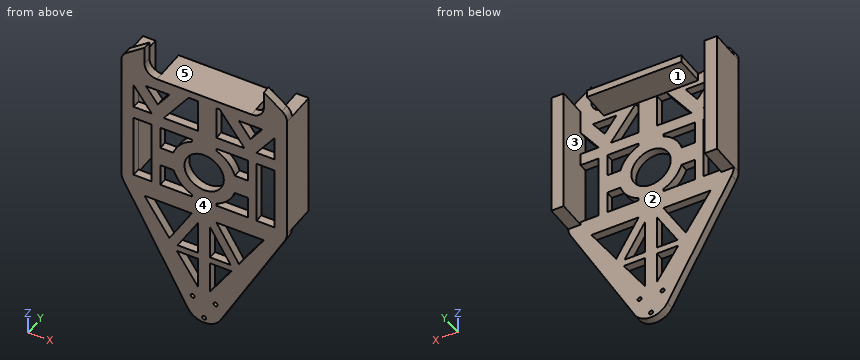
```python
from build123d import *

# Parameters (mm, degrees)
SKETCH1_R            = 47.5
BOSS_EXTRUDE6_DEPTH  = 20
FILLET2_R            = 30
SKETCH3_W            = 227.888974491
SKETCH3_H            = 17.82820952
SKETCH3_W_2          = 30.029703607
SKETCH3_H_2          = 306.819916415
SKETCH3_W_3          = 30
BOSS_EXTRUDE12_DEPTH = 70
FILLET3_R            = 45
FILLET4_R            = 45
SKETCH4_R            = 4.852465173
CUT_EXTRUDE2_DEPTH   = 21


with BuildPart() as part:
    # Sketch1 → Boss-Extrude6 (new body)
    with BuildSketch(Plane(origin=(0, 0, 0), x_dir=(1, 0, 0), z_dir=(0, 1, 0))):
        Polygon((-324.500042801, -72.630227613), (-324.500042801, 0), (-36.61106831, 0), (-36.61106831, -72.630227613), (19.444444444, -30.98937664), (19.444444444, 0), (19.444444444, 300), (-180.555555556, 662.976241067), (-380.555555556, 300), (-380.555555556, 0), (-380.555555556, -30.98937664), align=None)
        Polygon((-264.055692307, 30), (-320.898350202, 30), (-292.477021255, 68.259836918), align=None, mode=Mode.SUBTRACT)
        Polygon((-350.555555556, 40.384990781), (-350.555555556, 98.955926659), (-307.046121917, 98.955926659), align=None, mode=Mode.SUBTRACT)
        Polygon((-194.895952536, 18.381237109), (-218.052993309, 18.381237109), (-277.907920592, 98.955926659), (-194.895952536, 98.955926659), align=None, mode=Mode.SUBTRACT)
        Polygon((-307.046121917, 128.955926659), (-350.555555556, 128.955926659), (-350.555555556, 178.791030317), (-350.555555556, 221.457829656), (-350.555555556, 283.955926659), (-307.046121917, 283.955926659), (-307.046121917, 221.457829656), (-307.046121917, 178.791030317), align=None, mode=Mode.SUBTRACT)
        with BuildLine():
            Line((-210.32776095, 128.955926659), (-286.18247229, 128.955926659))
            Line((-286.18247229, 128.955926659), (-286.18247229, 183.722078004))
            Line((-286.18247229, 183.722078004), (-254.646190087, 183.722078004))
            ThreePointArc((-254.646190087, 183.722078004), (-237.937656941, 154.364234033), (-210.32776095, 134.902689235))
            Line((-210.32776095, 134.902689235), (-210.32776095, 128.955926659))
        make_face(mode=Mode.SUBTRACT)
        with BuildLine():
            Line((-286.18247229, 230.610640855), (-286.18247229, 283.955926659))
            Line((-286.18247229, 283.955926659), (-210.32776095, 283.955926659))
            Line((-210.32776095, 283.955926659), (-210.32776095, 278.009164084))
            ThreePointArc((-210.32776095, 278.009164084), (-237.43400989, 259.09708387), (-254.195217302, 230.610640855))
            Line((-254.195217302, 230.610640855), (-286.18247229, 230.610640855))
        make_face(mode=Mode.SUBTRACT)
        with Locations((-180.555555556, 206.455926659)):
            Circle(SKETCH1_R, mode=Mode.SUBTRACT)
        Polygon((-143.058117802, 18.381237109), (-150.783350161, 18.381237109), (-150.783350161, 98.955926659), (-83.203190519, 98.955926659), align=None, mode=Mode.SUBTRACT)
        Polygon((-68.634089856, 68.259836918), (-40.212760909, 30), (-97.055418804, 30), align=None, mode=Mode.SUBTRACT)
        Polygon((-10.555555556, 98.955926659), (-10.555555556, 40.384990781), (-54.064989194, 98.955926659), align=None, mode=Mode.SUBTRACT)
        with BuildLine():
            Line((-150.783350161, 128.955926659), (-150.783350161, 134.902689235))
            ThreePointArc((-150.783350161, 134.902689235), (-123.17345417, 154.364234033), (-106.464921024, 183.722078004))
            Line((-106.464921024, 183.722078004), (-74.928638821, 183.722078004))
            Line((-74.928638821, 183.722078004), (-74.928638821, 128.955926659))
            Line((-74.928638821, 128.955926659), (-150.783350161, 128.955926659))
        make_face(mode=Mode.SUBTRACT)
        with BuildLine():
            ThreePointArc((-106.915893809, 230.610640855), (-123.677101221, 259.09708387), (-150.783350161, 278.009164084))
            Line((-150.783350161, 278.009164084), (-150.783350161, 283.955926659))
            Line((-150.783350161, 283.955926659), (-74.928638821, 283.955926659))
            Line((-74.928638821, 283.955926659), (-74.928638821, 230.610640855))
            Line((-74.928638821, 230.610640855), (-106.915893809, 230.610640855))
        make_face(mode=Mode.SUBTRACT)
        Polygon((-10.555555556, 178.791030317), (-10.555555556, 128.955926659), (-54.064989194, 128.955926659), (-54.064989194, 178.791030317), (-54.064989194, 221.457829656), (-54.064989194, 283.955926659), (-10.555555556, 283.955926659), (-10.555555556, 221.457829656), align=None, mode=Mode.SUBTRACT)
        Polygon((-210.32776095, 330), (-324.500042801, 330), (-264.477795432, 420.033371054), align=None, mode=Mode.SUBTRACT)
        Polygon((-194.895952536, 348.542048906), (-244.539447118, 431.082553467), (-194.895952536, 431.082553467), align=None, mode=Mode.SUBTRACT)
        Polygon((-246.308768225, 447.286911864), (-194.895952536, 524.406135398), (-194.895952536, 447.286911864), align=None, mode=Mode.SUBTRACT)
        Polygon((-96.633315679, 420.033371054), (-36.61106831, 330), (-150.783350161, 330), align=None, mode=Mode.SUBTRACT)
        Polygon((-166.215158575, 431.082553467), (-116.571663993, 431.082553467), (-166.215158575, 348.542048906), align=None, mode=Mode.SUBTRACT)
        Polygon((-166.215158575, 524.406135398), (-114.802342886, 447.286911864), (-166.215158575, 447.286911864), align=None, mode=Mode.SUBTRACT)
    extrude(amount=BOSS_EXTRUDE6_DEPTH)

    # Fillet2
    fillet2_edges = [part.edges().sort_by_distance(p)[0] for p in [
        (19.444444444, 10, 30.98937664),
        (-36.61106831, 10, 0),
        (-324.500042801, 10, 0),
        (-380.555555556, 10, 30.98937664),
    ]]
    fillet(fillet2_edges, radius=FILLET2_R)

    # Sketch3 → Boss-Extrude12 (add)
    with BuildSketch(Plane(origin=(0, 20, 0), x_dir=(1, 0, 0), z_dir=(0, 1, 0))):
        with Locations((-180.555555556, 8.91410476)):
            Rectangle(SKETCH3_W, SKETCH3_H)
        with Locations((-365.540703753, 137.50677266)):
            Rectangle(SKETCH3_W_2, SKETCH3_H_2)
        with Locations((4.444444444, 137.50677266)):
            Rectangle(SKETCH3_W_3, SKETCH3_H_2)
    extrude(amount=BOSS_EXTRUDE12_DEPTH)

    # Fillet3
    fillet3_edges = [part.edges().sort_by_distance(p)[0] for p in [
        (-180.555555556, 10, -662.976241067),
    ]]
    fillet(fillet3_edges, radius=FILLET3_R)

    # Fillet4
    fillet4_edges = [part.edges().sort_by_distance(p)[0] for p in [
        (-380.555555556, 10, -300),
        (19.444444444, 10, -300),
    ]]
    fillet(fillet4_edges, radius=FILLET4_R)

    # Sketch4 → Cut-Extrude2 (cut, through all)
    with BuildSketch(Plane(origin=(0, 20, 0), x_dir=(1, 0, 0), z_dir=(0, 1, 0))):
        with Locations((-180.555555556, 601.729619553)):
            Circle(SKETCH4_R)
        with Locations((-208.268368477, 553.729619553)):
            Circle(SKETCH4_R)
        with Locations((-152.842742634, 553.729619553)):
            Circle(SKETCH4_R)
    extrude(amount=-CUT_EXTRUDE2_DEPTH, mode=Mode.SUBTRACT)


solid = part.part
```
The listing builds one solid part. Answer for the finished solid, in the listing's coordinates (mm). Face numbers are marked on the shaded views. A direction names the side the tool comes from. Give positions to 0.01 mm unless a question says otherwise; leave off trailing zeros. Order: outer loops, then holes, each group sorted by start corner. A loop starts at its lowest first (then second) coordinate and runs counter-clockwise, first axis right, second up. Notation, with made-up numbers: (-1, 31.25) - (39, 31.25) arc R28 ccw to (39, 52.25) - close; hole circle Ø1 at (52.5, 25.5). An arc over 180 degrees is marked (long way). Answer in a Markdown table with one row per item. Add a question column.
Q1. Which of the six approach directions +Z, -Z, +X, -X, +Y, -Y give full straight-line access (tool end or side, diameter ignored) to the marked faces 4 and 5?
Q2. The part is cut by section B-B (z = -486.5). Determine the outline of the cut face in (x, y).
Q3. For a pull along Z with two mould halves and no side action, classify the marked faces 1, 2 and 3 as released by +Z, released by -Z, zero draft, split by the parting line, or undercut.
Q4. Find the intervals of material crossed by line 1 along X through (y, z) = (43, -267.5); line 2 along Z through (x, y) = (-246, 18.5); line 3 along X through (y, z) = (8, -403), in increasing order. Write a range as [from, to].
Q5. Given P1, Ø6, axis at y = 9.5, z = -410, coming from the +X side; P2, Ø16, axis at x = -333.5, y = 14, coming from the -Z side; P3, Ø6, axis at x = -291.5, y = 11, coming from the -Z side, each flat-ended and moving along its own axis, determine where each tip first touches the part or whether it passes through.
Q6. The part is cut by section A-A (y = 70). Determine the outline of the cut face in (x, z).
Q7. The part is cut by section C-C (z = -192). Give the number of separate pieces and of enclosed holes in the cut face, then the cut area to 3 significant figures.
Determined:
| question | item | result |
|---|---|---|
| 1 | face 4 | +Z, -Z, +X, -X, -Y |
| 1 | face 5 | +Z, +Y, -Y |
| 2 | outline | (-277.79, 0) - (-220.17, 0) - (-220.17, 20) - (-277.79, 20) - close; (-194.9, 0) - (-166.22, 0) - (-166.22, 20) - (-194.9, 20) - close; (-140.94, 0) - (-83.32, 0) - (-83.32, 20) - (-140.94, 20) - close |
| 3 | face 1 | released by -Z |
| 3 | face 2 | zero draft |
| 3 | face 3 | undercut |
| 4 | line 1 | x = [-380.56, -350.53], [-10.56, 19.44] |
| 4 | line 2 | z = [-544.2, -447.75], [-447.29, -389.31], [-330, -283.96], [-247.97, -164.94], [-128.96, -98.96], [-56, 0] |
| 4 | line 3 | x = [-323.8, -275.83], [-254.23, -227.65], [-194.9, -166.22], [-133.46, -106.88], [-85.28, -37.31] |
| 5 | P1 | stops at x = -39.51 |
| 5 | P2 | stops at z = -399.92 |
| 5 | P3 | stops at z = -467.07 |
| 6 | outline | (-380.56, -288.42) arc R45 ccw to (-380.49, -290.92) - (-350.53, -290.92) - (-350.53, 15.9) - (-380.56, 15.9) - close; (-294.5, -17.83) - (-66.61, -17.83) - (-66.61, 0) - (-294.5, 0) - close; (-10.56, -290.92) - (19.38, -290.92) arc R45 ccw to (19.44, -288.42) - (19.44, 15.9) - (-10.56, 15.9) - close |
| 7 | separate pieces | 4 |
| 7 | enclosed holes | 0 |
| 7 | area | 8,650 mm² |
